```python
from build123d import *

# Parameters (mm, degrees)
F0_W     = 30
F0_H     = 30
F1_DEPTH = 30
F3_DEPTH = 30.001
F5_R     = 5
F6_SIZE  = 5


with BuildPart() as f1:
    # F0 (on Top) → F1 (new body)
    with BuildSketch(Plane.XY):
        Rectangle(F0_W, F0_H)
    extrude(amount=F1_DEPTH)

    # F2 (on face) → F3 (cut, through all)
    with BuildSketch(Plane.XZ.offset(15)):
        with BuildLine():
            ThreePointArc((0, 20), (-3.5355339059, 11.4644660941), (5, 15))
            ThreePointArc((5, 15), (3.5355339059, 18.5355339059), (0, 20))
        make_face()
    extrude(amount=-F3_DEPTH, mode=Mode.SUBTRACT)

    # F4: F1 across face


with BuildPart() as f1_1:
    add(f1.part)
    add(f1.part.mirror(Plane(origin=(15, 0, 15), x_dir=(0, 1, 0), z_dir=(1, 0, 0))))

    # F5
    f5_edges = [f1_1.edges().sort_by_distance(p)[0] for p in [
        (45, -15, 15),
    ]]
    fillet(f5_edges, radius=F5_R)

    # F6
    f6_edges = [f1_1.edges().sort_by_distance(p)[0] for p in [
        (45, 15, 15),
    ]]
    chamfer(f6_edges, length=F6_SIZE)


solid = f1_1.part
```
Verification items for the finished model (mm, model axes). Give positions to 0.01 mm unless a question says otherwise; leave off trailing zeros. Loops run counter-clockwise (first coordinate to the right, second up) from the corner with the lowest first, then second, coordinate; pieces in that order, holes last. Notation, with made-up numbers: M 80,66 L 139,66 A33 cw 139,103 Z; hole C 69,-39.75 d3. An arc over 180 degrees is marked long. One line per question, with ' | ' between items.
Item 1: Thickness scan on line 1 (X direction, y = -1, z = 15); line 2 (X direction, y = 8.75, z = 13); line 3 (Z direction, x = 30, y = 0.5). Record the ranges inside material, lowest first. Write a range as [from, to].
Completed:
line 1: x = [-15, -5], [5, 25], [35, 45] | line 2: x = [-15, -4.58], [4.58, 25.42], [34.58, 45] | line 3: z = [0, 10], [20, 30]
Item 2: Depth check by flat-ended pin: P1, Ø9, axis at x = 30, z = 15, coming from the +Y side. Enter the tip coordinate at first touch or a pass-through.
Completed:
P1: passes through
Item 3: Section check B-B, the plane z = 11.5. Record the cut outline in (x, y), plus the area to 3 significant figures.
Completed:
outline: M -15,-15 L -3.57,-15 L -3.57,15 L -15,15 Z; M 3.57,-15 L 26.43,-15 L 26.43,15 L 3.57,15 Z; M 33.57,-15 L 40,-15 A5 ccw 45,-10 L 45,10 L 40,15 L 33.57,15 Z | area: 1,350 mm^2
Item 4: Section check A-A, the plane y = 6. Record the cut outline in (x, z).
Completed:
outline: M -15,0 L 45,0 L 45,30 L -15,30 Z; hole C 0,15 d10; hole C 30,15 d10
